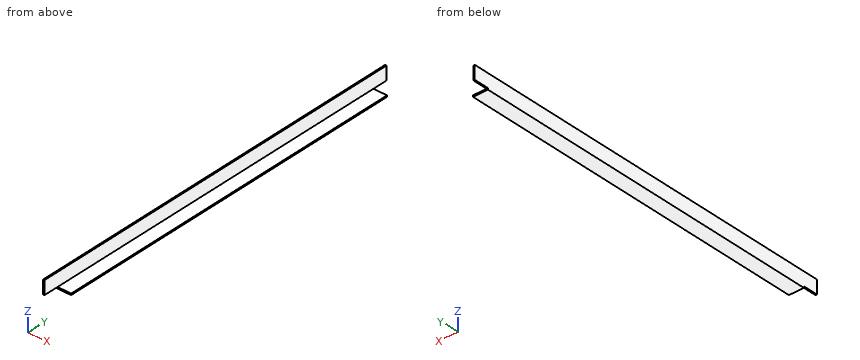
```python
from build123d import *

# Parameters (mm, degrees)
F1_DEPTH = 660.4
F2_W     = 50.8
F2_H     = 50.8
F3_DEPTH = 4.7625


with BuildPart() as f1:
    # F0 (on Front) → F1 (new body, symmetric)
    with BuildSketch(Plane.XZ):
        Polygon((0, 50.8), (0, 0), (50.8, 0), (50.8, 4.7625), (4.7625, 4.7625), (4.7625, 50.8), align=None)
    extrude(amount=F1_DEPTH, both=True)

    # F2 (on face) → F3 (cut, through all)
    with BuildSketch(Plane(origin=(0, 0, 0), x_dir=(1, 0, 0), z_dir=(0, 0, -1))):
        with Locations((25.4, 635)):
            Rectangle(F2_W, F2_H)
        with Locations((25.4, -635)):
            Rectangle(F2_W, F2_H)
    extrude(amount=-F3_DEPTH, mode=Mode.SUBTRACT)


solid = f1.part
```
Build history of the part. All positions in model axes, mm. Give positions to 0.01 mm unless a question says otherwise; leave off trailing zeros. Loops run counter-clockwise (first coordinate to the right, second up) from the corner with the lowest first, then second, coordinate; pieces in that order, holes last. Notation, with made-up numbers: (18, -12) - (55, -12) arc R21 ccw to (55, 6) - close; hole circle Ø8 at (24, -16.75). An arc over 180 degrees is marked (long way). Use a Markdown table: item, result.
(1) Band-saw the part on A-A (y = -229.5). Give the cut face in (x, z).
Taken from the geometry:
| item | result |
|---|---|
| outline | (0, 0) - (50.8, 0) - (50.8, 4.76) - (4.76, 4.76) - (4.76, 50.8) - (0, 50.8) - close |
(2) Band-saw the part on B-B (x = 34). Give the cut face in (y, z), and give its area (3 significant figures).
Taken from the geometry:
| item | result |
|---|---|
| outline | (-609.6, 0) - (609.6, 0) - (609.6, 4.76) - (-609.6, 4.76) - close |
| area | 5,810 mm2 |
(3) Wall check: line 1 along Z through (x, y) = (46, -606.5); line 2 along Y through (x, z) = (47.5, 4). Give the ranges that are in metal, low to high.
Taken from the geometry:
| item | result |
|---|---|
| line 1 | 0 to 4.76 |
| line 2 | -609.6 to 609.6 |
(4) Band-saw the part on C-C (z = 27). Give the cut face in (x, y).
Taken from the geometry:
| item | result |
|---|---|
| outline | (0, -660.4) - (4.76, -660.4) - (4.76, 660.4) - (0, 660.4) - close |
(5) Drop flat-ended pins along their axis: pin 1 Ø1.4 at (x, y) = (2, 638) entering from -Z; pin 2 Ø4 at (x, y) = (40.5, 376.5) entering from +Z; pin 3 Ø3 at (y, z) = (268.5, 5.5) entering from +X; pin 4 Ø4 at (x, z) = (31, 3) entering from -Y. Give the stop position or say it passes through.
Taken from the geometry:
| item | result |
|---|---|
| pin 1 | z = 4.76 |
| pin 2 | z = 4.76 |
| pin 3 | x = 50.8 |
| pin 4 | y = -609.6 |
